The listing builds one solid part. Answer for the finished solid, in the listing's coordinates (mm). Face numbers are marked on the shaded views. A direction names the side the tool comes from. Coordinates: 2 decimals unless noted, no trailing zeros. Write each loop counter-clockwise with the first axis right and the second up, starting at its lowest first coordinate (ties: lowest second). Pieces come first, ordered by that corner, then holes.
(1) The part is cut by section C-C on x = 107.5. Determine the outline of the cut face in (y, z), plus the area to 3 significant figures.
(2) Which of the six approach directions +Z, -Z, +X, -X, +Y, -Y give full straight-line access (tool end or side, diameter ignored) to the marked faces 1 and 2?
(3) The part is cut by section A-A on y = 0. Determine the outline of the cut face in (x, z).
(4) The part is cut by section D-D on z = 12. Determine the outline of the cut face in (x, y), plus the area to 3 significant figures.
(5) Straight lines are drawn through the part: line 1 (Z direction, x = 44, y = 0.5); line 2 (X direction, y = -3.5, z = 12.5). For each, find the intervals that lie inside material, in ascending order.
(6) Given P1, Ø12, axis at x = 84, y = 5, coming from the +Z side; P2, Ø12, axis at x = 143.5, z = 7, coming from the -Y side; P3, Ø1.5, axis at x = 141, z = -6.5, coming from the -Y side, each flat-ended and moving along its own axis, determine where each tip first touches the part or whether it passes through.
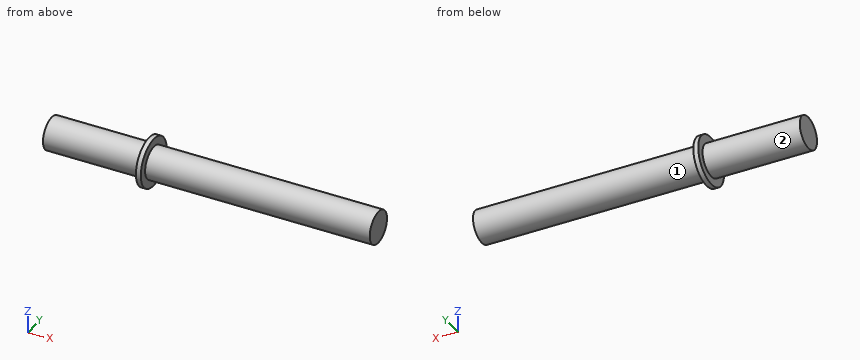
from build123d import *

# Parameters (mm, degrees)
CROQUIS1_R              = 10
SALIENTE_EXTRUIR1_DEPTH = 200
CROQUIS2_R              = 15
SALIENTE_EXTRUIR2_DEPTH = 3


with BuildPart() as part:
    # Croquis1 → Saliente-Extruir1 (new body)
    with BuildSketch(Plane(origin=(0, 0, 0), x_dir=(0, 0, -1), z_dir=(1, 0, 0))):
        Circle(CROQUIS1_R)
    extrude(amount=SALIENTE_EXTRUIR1_DEPTH)

    # Croquis2 → Saliente-Extruir2 (add)
    with BuildSketch(Plane.ZY.offset(-62.5)):
        Circle(CROQUIS2_R)
    extrude(amount=SALIENTE_EXTRUIR2_DEPTH)


solid = part.part
Model answer:
1. outline: circle Ø20 at (0, 0)
1. area: 314 mm2
2. face 1: +X
2. face 2: -X
3. outline: (0, -10) - (59.5, -10) - (59.5, -15) - (62.5, -15) - (62.5, -10) - (200, -10) - (200, 10) - (62.5, 10) - (62.5, 15) - (59.5, 15) - (59.5, 10) - (0, 10) - close
4. outline: (59.5, -9) - (62.5, -9) - (62.5, 9) - (59.5, 9) - close
4. area: 54.0 mm2
5. line 1: z = -9.99 to 9.99
5. line 2: x = 59.5 to 62.5
6. P1: stops at z = 10
6. P2: stops at y = -9.95
6. P3: stops at y = -8.18
